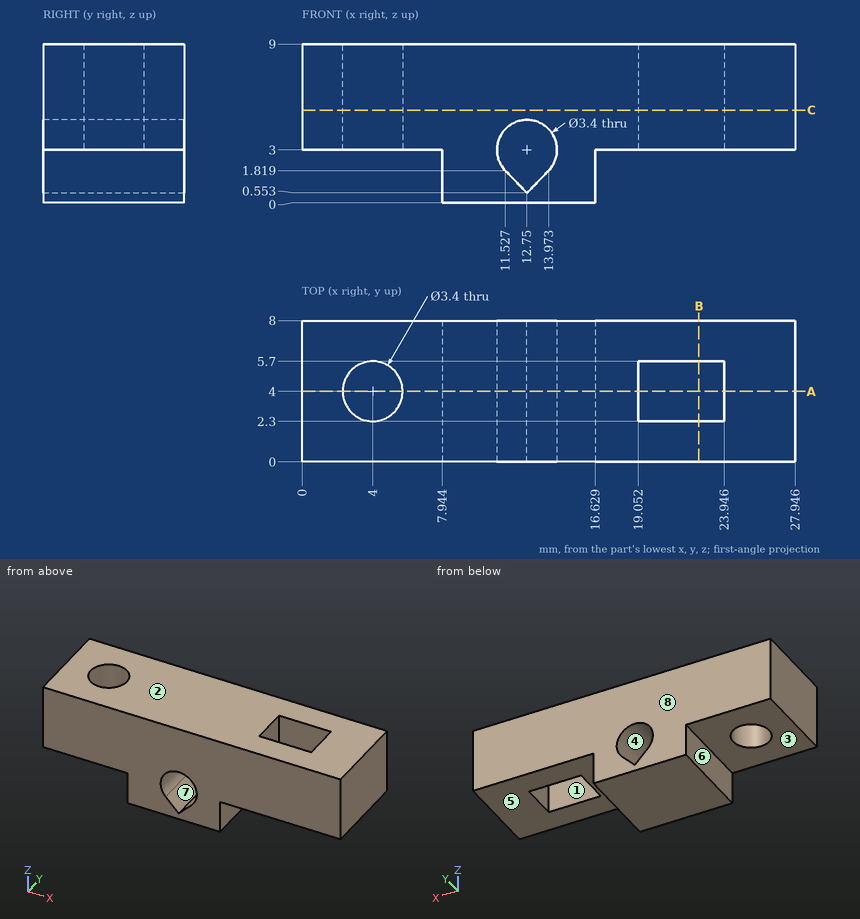
Geometry check sheet. Reference: drawing and pictorial views, mm from the part's lowest x, y, z. A direction names the side the tool comes from. Give positions to 0.01 mm unless a question says otherwise; leave off trailing zeros. Order: outer loops, then holes, each group sorted by start corner. A loop starts at its lowest first (then second) coordinate and runs counter-clockwise, first axis right, second up. Notation, with made-up numbers: (77, 75) -> (108, 75) arc R20 cw to (108, 99) -> close; hole circle Ø7 at (33.25, 11.5). An arc over 180 degrees is marked (long way). Use CSV: the item, a comma, the result in double quotes. Start each with the question number.
1) Sectioned sample at C-C, the plane z = 5.25. Record the boundary of the cut face in (x, y) (1 decimal), plus the area to 3 significant figures.
2) Sectioned sample at A-A, the plane y = 4. Give the number of separate pieces and of enclosed holes in the cut face, plus the area to 3 significant figures.
3) Material ranges on line 1 (Y direction, x = 4, z = 5.2); line 2 (X direction, y = 2, z = 3.25) (1 decimal); line 3 (Y direction, x = 5.5, z = 6), recorded low to high. Write a range as from..to.
4) Go/stop test with flat-tipped pins: P1, Ø4, axis at x = 21.5, y = 5.5, coming from the -Z side; P2, Ø1.5, axis at y = 1.5, z = 1.5, coming from the -X side; P3, Ø3.5, axis at y = 2, z = 2, coming from the -X side; P4, Ø1.5, axis at y = 3.5, z = 1, coming from the +X side. Record where each tip stops, or that it passes through.
5) Sectioned sample at B-B, the plane x = 22.5. Record the boundary of the cut face in (y, z), plus the area to 3 significant figures.
6) Mould release check, pull along X, two halves, no side actions. Record for the marked faces 6, 7 and 8: released by +X, released by -X, zero draft, split by the parting line, or undercut.
7) Set-up check for the marked faces 1, 2, 3, 4 and 5: record each of +Z, -Z, +X, -X, +Y, -Y from which the full face is reachable in a straight line by a thin tool's end or side.
Recorded:
1,outline,"(0, 0) -> (27.9, 0) -> (27.9, 8) -> (0, 8) -> close; hole circle Ø3.4 at (4, 4); hole (19.1, 2.3) -> (23.9, 2.3) -> (23.9, 5.7) -> (19.1, 5.7) -> close"
1,area,"198 mm2"
2,separate pieces,"3"
2,enclosed holes,"1"
2,area,"134 mm2"
3,line 1,"0..2.3, 5.7..8"
3,line 2,"0..11.1, 14.4..27.9"
3,line 3,"0..3.2, 4.8..8"
4,P1,"z = 3"
4,P2,"x = 7.94"
4,P3,"x = 0"
4,P4,"x = 16.63"
5,outline,"(0, 3) -> (2.3, 3) -> (2.3, 9) -> (0, 9) -> close; (5.7, 3) -> (8, 3) -> (8, 9) -> (5.7, 9) -> close"
5,area,"27.6 mm2"
6,face 6,"released by -X"
6,face 7,"undercut"
6,face 8,"zero draft"
7,face 1,"+Z, -Z"
7,face 2,"+Z, +X, -X, +Y, -Y"
7,face 3,"-Z, -X, +Y, -Y"
7,face 4,"+Y, -Y"
7,face 5,"-Z, +X, +Y, -Y"
